Part model, mm, in its own coordinate system. Give positions to 0.01 mm unless a question says otherwise; leave off trailing zeros. Order: outer loops, then holes, each group sorted by start corner. A loop starts at its lowest first (then second) coordinate and runs counter-clockwise, first axis right, second up. Notation, with made-up numbers: (56, 51) -> (112, 51) arc R36 cw to (112, 89) -> close; hole circle Ø2 at (66.5, 53). An arc over 180 degrees is marked (long way). Write item = value, one per line. Start each with the question number.
(1) Saw through at B-B, the plane z = 36. List the corners of the cut face in (x, y), then the cut area to 3 significant figures.
(2) Saw through at A-A, the plane x = -99.5. List the corners of the cut face in (y, z), then the cut area to 3 significant figures.
(3) Saw through at D-D, the plane z = 85.5. List the corners of the cut face in (x, y), then the cut area to 3 significant figures.
(4) Probe line 1 along Z through (x, y) = (6.5, 2.1); line 2 along X through (y, z) = (2.7, 17.5); line 3 along X through (y, z) = (2.9, 44). List the from-to ranges inside material, lowest first. Write a range as from..to.
(5) Saw through at C-C, the plane y = 2.2. State how many separate pieces and enclosed holes the cut face has, then the cut area to 3 significant figures.
from build123d import *

# Parameters (mm, degrees)
SKETCH1_W             = 368.3
SKETCH1_H             = 228.6
BOSS_EXTRUDE1_DEPTH   = 4.7625
CUT_EXTRUDE1_DEPTH    = 217.791129676
SKETCH_PATTERN1_DEPTH = 4.7625
FILLET1_R             = 2.54


# Read off the part's stored shape, not the designer's step: Sketch-Pattern1
with BuildPart() as part:
    # Sketch1 → Boss-Extrude1 (new body)
    with BuildSketch(Plane(origin=(0, 0, 0), x_dir=(1, 0, 0), z_dir=(0, 1, 0))):
        Rectangle(SKETCH1_W, SKETCH1_H)
    extrude(amount=BOSS_EXTRUDE1_DEPTH)

    # Sketch3 → Cut-Extrude1 (cut, through all)
    with BuildSketch(Plane.XZ):
        with BuildLine():
            Line((143.533374481, -3.245454654), (95.226625519, -3.245454654))
            ThreePointArc((95.226625519, -3.245454654), (63.594954654, -53.5305), (95.226625519, -103.815545346))
            Line((95.226625519, -103.815545346), (143.533374481, -103.815545346))
            ThreePointArc((143.533374481, -103.815545346), (175.165045346, -53.5305), (143.533374481, -3.245454654))
        make_face()
    extrude(amount=-CUT_EXTRUDE1_DEPTH, mode=Mode.SUBTRACT)

    # Sketch-Pattern1 outline → Sketch-Pattern1 (cut)
    with BuildSketch(Plane(origin=(0, 0, 0), x_dir=(1, 0, 0), z_dir=(0, 1, 0))):
        with BuildLine():
            ThreePointArc((-24.153374481, 103.815545346), (-55.785045346, 53.5305), (-24.153374481, 3.245454654))
            Line((-24.153374481, 3.245454654), (24.153374481, 3.245454654))
            ThreePointArc((24.153374481, 3.245454654), (55.785045346, 53.5305), (24.153374481, 103.815545346))
            Line((24.153374481, 103.815545346), (-24.153374481, 103.815545346))
        make_face()
        with BuildLine():
            ThreePointArc((-143.533374481, 103.815545346), (-175.165045346, 53.5305), (-143.533374481, 3.245454654))
            Line((-143.533374481, 3.245454654), (-95.226625519, 3.245454654))
            ThreePointArc((-95.226625519, 3.245454654), (-63.594954654, 53.5305), (-95.226625519, 103.815545346))
            Line((-95.226625519, 103.815545346), (-143.533374481, 103.815545346))
        make_face()
        with BuildLine():
            ThreePointArc((95.226625519, -3.245454654), (63.594954654, -53.5305), (95.226625519, -103.815545346))
            Line((95.226625519, -103.815545346), (143.533374481, -103.815545346))
            ThreePointArc((143.533374481, -103.815545346), (175.165045346, -53.5305), (143.533374481, -3.245454654))
            Line((143.533374481, -3.245454654), (95.226625519, -3.245454654))
        make_face()
        with BuildLine():
            ThreePointArc((-24.153374481, -3.245454654), (-55.785045346, -53.5305), (-24.153374481, -103.815545346))
            Line((-24.153374481, -103.815545346), (24.153374481, -103.815545346))
            ThreePointArc((24.153374481, -103.815545346), (55.785045346, -53.5305), (24.153374481, -3.245454654))
            Line((24.153374481, -3.245454654), (-24.153374481, -3.245454654))
        make_face()
        with BuildLine():
            ThreePointArc((-143.533374481, -3.245454654), (-175.165045346, -53.5305), (-143.533374481, -103.815545346))
            Line((-143.533374481, -103.815545346), (-95.226625519, -103.815545346))
            ThreePointArc((-95.226625519, -103.815545346), (-63.594954654, -53.5305), (-95.226625519, -3.245454654))
            Line((-95.226625519, -3.245454654), (-143.533374481, -3.245454654))
        make_face()
    extrude(amount=SKETCH_PATTERN1_DEPTH, mode=Mode.SUBTRACT)

    # Fillet1
    fillet1_edges = [part.edges().sort_by_distance(p)[0] for p in [
        (184.15, 2.38125, 114.3),
        (-184.15, 2.38125, 114.3),
        (-184.15, 2.38125, -114.3),
        (184.15, 2.38125, -114.3),
    ]]
    fillet(fillet1_edges, radius=FILLET1_R)


solid = part.part
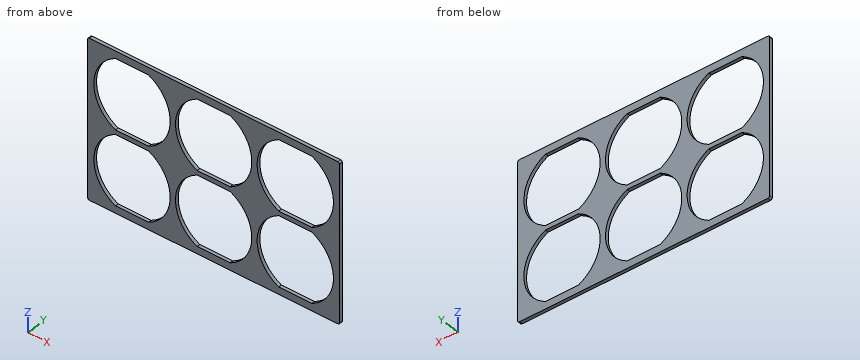
Results list:
q1.outline = (-184.15, 0) -> (-172.34, 0) -> (-172.34, 4.76) -> (-184.15, 4.76) -> close; (-66.42, 0) -> (-52.96, 0) -> (-52.96, 4.76) -> (-66.42, 4.76) -> close; (52.96, 0) -> (66.42, 0) -> (66.42, 4.76) -> (52.96, 4.76) -> close; (172.34, 0) -> (184.15, 0) -> (184.15, 4.76) -> (172.34, 4.76) -> close
q1.area = 241 mm^2
q2.outline = (0, -114.3) -> (4.76, -114.3) -> (4.76, -103.82) -> (0, -103.82) -> close; (0, -3.25) -> (4.76, -3.25) -> (4.76, 3.25) -> (0, 3.25) -> close; (0, 103.82) -> (4.76, 103.82) -> (4.76, 114.3) -> (0, 114.3) -> close
q2.area = 131 mm^2
q3.outline = (-184.15, 0) -> (-165.1, 0) -> (-165.1, 4.76) -> (-184.15, 4.76) -> close; (-73.66, 0) -> (-45.72, 0) -> (-45.72, 4.76) -> (-73.66, 4.76) -> close; (45.72, 0) -> (73.66, 0) -> (73.66, 4.76) -> (45.72, 4.76) -> close; (165.1, 0) -> (184.15, 0) -> (184.15, 4.76) -> (165.1, 4.76) -> close
q3.area = 448 mm^2
q4.line_1 = -114.3..-103.82, -3.25..3.25, 103.82..114.3
q4.line_2 = -184.15..-161.97, -76.79..-42.59, 42.59..76.79, 161.97..184.15
q4.line_3 = -184.15..-174.34, -64.42..-54.96, 54.96..64.42, 174.34..184.15
q5.separate_pieces = 1
q5.enclosed_holes = 6
q5.area = 27,700 mm^2
